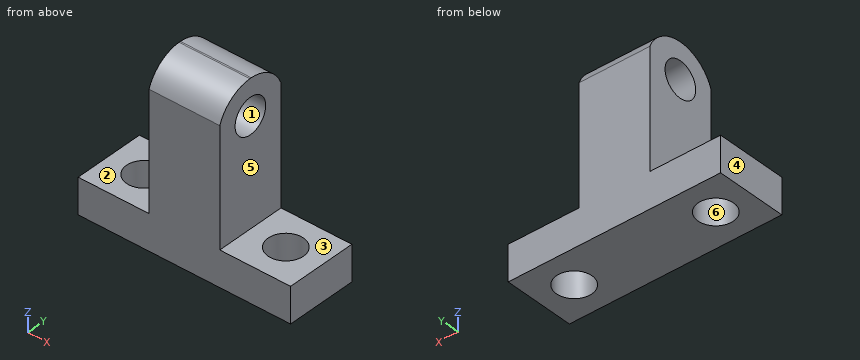
```python
from build123d import *

# Parameters (mm, degrees)
F0_W      = 76.2
F0_H      = 63.5
F1_DEPTH  = 25.4
F2_W      = 25.4
F2_H      = 50.8
F3_DEPTH  = 25.401
F7_DEPTH  = 25.4
F5_R      = 6.35
F4_R      = 6.35
F8_DEPTH  = 25.4
F9_R      = 6.35
F10_DEPTH = 50.801


with BuildPart() as f1:
    # F0 (on Front) → F1 (new body)
    with BuildSketch(Plane.XZ):
        with Locations((-30.763134826, 27.8038036936)):
            Rectangle(F0_W, F0_H)
    extrude(amount=F1_DEPTH)

    # F2 (on face) → F3 (cut, through all)
    with BuildSketch(Plane.XZ.offset(25.4)):
        with Locations((-56.163134826, 34.1538036936)):
            Rectangle(F2_W, F2_H)
        with Locations((-5.363134826, 34.1538036936)):
            Rectangle(F2_W, F2_H)
    extrude(amount=-F3_DEPTH, mode=Mode.SUBTRACT)

    # F6 (on face) → F7 (cut)
    with BuildSketch(Plane.YZ.offset(-18.063134826)):
        with BuildLine():
            ThreePointArc((-25.4, 50.7014505565), (-20.5266979075, 57.0452252376), (-12.9306736435, 59.5538036936))
            Line((-12.9306736435, 59.5538036936), (-25.4, 59.5538036936))
            Line((-25.4, 59.5538036936), (-25.4, 50.7014505565))
        make_face()
        with BuildLine():
            ThreePointArc((-12.3705876013, 59.5538036936), (-4.8872224378, 57.1243511626), (0, 50.9584732354))
            Line((0, 50.9584732354), (0, 59.5538036936))
            Line((0, 59.5538036936), (-12.3705876013, 59.5538036936))
        make_face()
    extrude(amount=-F7_DEPTH, mode=Mode.SUBTRACT)

    # F5 (on face) + F4 (on face) → F8 (cut)
    with BuildSketch(Plane.XY.offset(8.7538036936)):
        with Locations((-5.363134826, -12.7)):
            Circle(F5_R)
    with BuildSketch(Plane.XY.offset(8.7538036936)):
        with Locations((-56.163134826, -12.7)):
            Circle(F4_R)
    extrude(amount=-F8_DEPTH, mode=Mode.SUBTRACT)

    # F9 (on face) → F10 (cut, through all)
    with BuildSketch(Plane.YZ.offset(-18.063134826)):
        with Locations((-12.7, 46.8580765592)):
            Circle(F9_R)
    extrude(amount=-F10_DEPTH, mode=Mode.SUBTRACT)


solid = f1.part
```
Can you work these out from the model? Positions are in its coordinate system, mm. Face numbers are marked on the shaded views. A direction names the side the tool comes from. Coordinates: 2 decimals unless noted, no trailing zeros. Write each loop counter-clockwise with the first axis right and the second up, starting at its lowest first coordinate (ties: lowest second). Pieces come first, ordered by that corner, then holes. Notation, with made-up numbers: M -25,27.5 L -8,27.5 A19 ccw -8,53.5 Z; hole C -2.75,-21 d4. An arc over 180 degrees is marked long. Answer as CSV lines item,"result".
Item 1: Imagine slicing it at D-D on z = 33.5. List the corners of the cut face in (x, y) for me.
Geometry results:
outline,"M -43.46,-25.4 L -18.06,-25.4 L -18.06,0 L -43.46,0 Z"
Item 2: Imagine slicing it at B-B on y = -17.5. List the corners of the cut face in (x, z) for me.
Geometry results:
outline,"M -68.86,-3.95 L -60.32,-3.95 L -60.32,8.75 L -68.86,8.75 Z; M -52.01,-3.95 L -9.52,-3.95 L -9.52,8.75 L -18.06,8.75 L -18.06,42.7 L -43.46,42.7 L -43.46,8.75 L -52.01,8.75 Z; M -43.46,51.02 L -18.06,51.02 L -18.06,58.66 L -43.46,58.66 Z; M -1.21,-3.95 L 7.34,-3.95 L 7.34,8.75 L -1.21,8.75 Z"
Item 3: Imagine slicing it at C-C on x = -24. List the corners of the cut face in (y, z) for me.
Geometry results:
outline,"M -25.4,-3.95 L 0,-3.95 L 0,50.96 A13.61 ccw -12.37,59.55 L -12.93,59.55 A13.61 ccw -25.4,50.7 Z; hole C -12.7,46.86 d12.7"
Item 4: We'd pull the mould along X, two halves only. Please class the marked faces 3, 4, 5 and 6: +X half, -X half, draft (parallel to the pull), parting line (faces both ways), or undercut.
Geometry results:
face 3,"draft"
face 4,"-X half"
face 5,"+X half"
face 6,"undercut"
Item 5: Imagine slicing it at A-A on x = -61. List the corners of the cut face in (y, z) for me, plus the area to 3 significant figures.
Geometry results:
outline,"M -25.4,-3.95 L -16.81,-3.95 L -16.81,8.75 L -25.4,8.75 Z; M -8.59,-3.95 L 0,-3.95 L 0,8.75 L -8.59,8.75 Z"
area,"218 mm2"
Item 6: I'm going to push flat-ended pins straight in: P1, Ø12.5, axis at y = -11, z = 32.5, coming from the -X side; P2, Ø3, axis at y = -21.5, z = 25.5, coming from the +X side; P3, Ø1, axis at x = -48, y = -12.5, coming from the +Z side. Where does each tip first touch, or does it pass through?
Geometry results:
P1,"stops at x = -43.46"
P2,"stops at x = -18.06"
P3,"stops at z = 8.75"
Item 7: On a 3-axis mill with a long thin cutter (end or side, diameter ignored), from which of +Z, -Z, +X, -X, +Y, -Y can I reach the whole of each face in a straight line? I mean the marked faces 1 and 2. Say none if no direction works.
Geometry results:
face 1,"+X, -X"
face 2,"+Z, -X, +Y, -Y"
Item 8: Please list where these lines run through material, in increasing order: line 1 along Z through (x, y) = (-29.5, -12.7); line 2 along X through (y, z) = (-23.5, 53); line 3 along Z through (x, y) = (2, -13).
Geometry results:
line 1,"z = -3.95 to 40.51, 53.21 to 59.55"
line 2,"x = -43.46 to -18.06"
line 3,"z = -3.95 to 8.75"
